Here's the drawing with two shaded views (mm, measured from the low corner). I have some questions. Coordinates: 2 decimals unless noted, no trailing zeros. Order: outer loops, then holes, each group sorted by start corner. A loop starts at its lowest first (then second) coordinate and runs counter-clockwise, first axis right, second up. Notation, with made-up numbers: (89, -8.75) - (102, -8.75) arc R35 ccw to (102, 27.25) - close; hole circle Ø10 at (21, 41). An arc over 180 degrees is marked (long way). Answer as CSV lines item,"result". Start each with the question number.
1. I need wall thicknesses on probe 1 along Y at (x, z) = (6, 100.5); probe 2 along Z at (x, y) = (11.5, 7). Which ranges of each line are inside material? Lowest first, please.
2. I want a section at A-A, the plane x = 6. List the corners of the cut face in (y, z) for me, and give its area (3 significant figures).
3. I want a section at C-C, the plane z = 73. List the corners of the cut face in (x, y) for me, and give its area (3 significant figures).
4. I want a section at B-B, the plane y = 6. List the corners of the cut face in (x, z) for me, and give its area (3 significant figures).
5. I want a section at D-D, the plane y = 10.5. List the corners of the cut face in (x, z) for me, and give its area (3 significant figures).
6. For pin 1 (1.5 mm diameter, centred on x = 5.5, z = 14, fed in from -Y); pin 2 (1.5 mm diameter, centred on x = 10.5, z = 19, fed in from -Y); pin 3 (1.5 mm diameter, centred on y = 7.5, z = 77, fed in from -X); pin 4 (1.5 mm diameter, centred on x = 4, z = 86.5, fed in from -Y), each with a flat end and sliding along its axis, tell me the tip position at first contact or that it passes through.
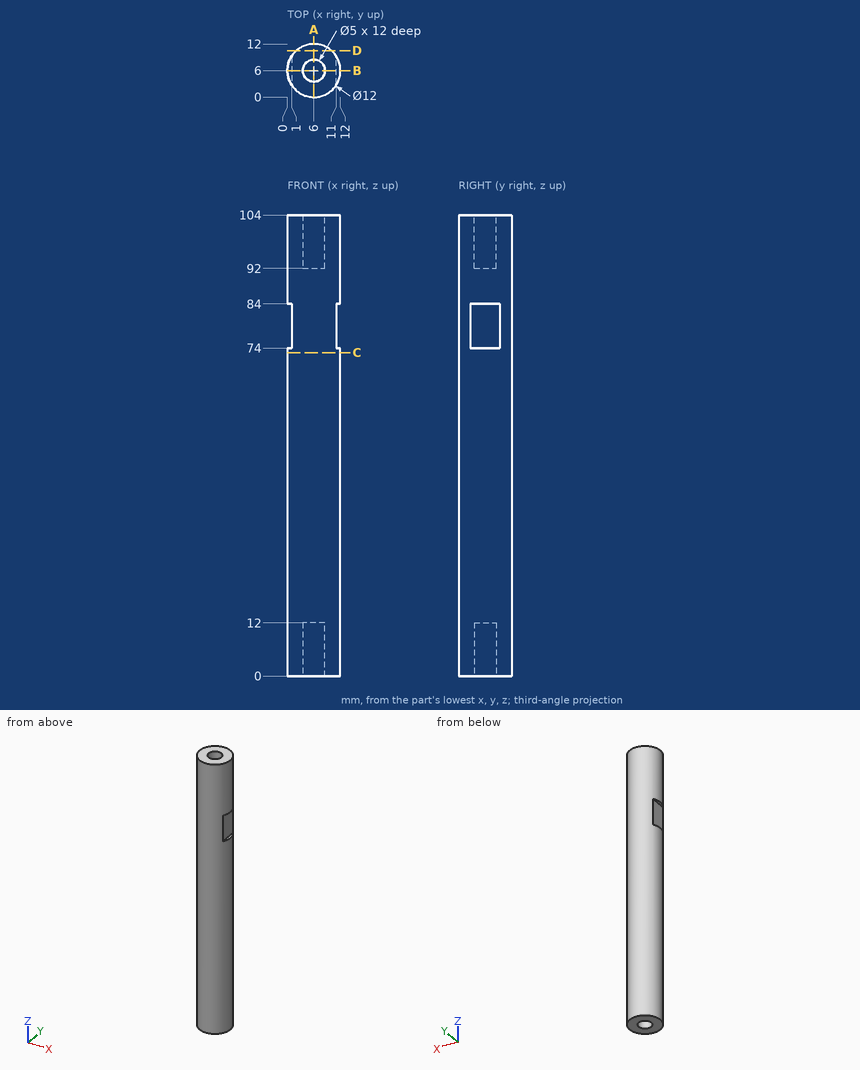
Solved:
1,probe 1,"y = 0 to 3.5, 8.5 to 12"
1,probe 2,"z = 0 to 74, 84 to 104"
2,outline,"(0, 0) - (3.5, 0) - (3.5, 12) - (8.5, 12) - (8.5, 0) - (12, 0) - (12, 104) - (8.5, 104) - (8.5, 92) - (3.5, 92) - (3.5, 104) - (0, 104) - close"
2,area,"1,130 mm2"
3,outline,"circle Ø12 at (6, 6)"
3,area,"113 mm2"
4,outline,"(0, 0) - (3.5, 0) - (3.5, 12) - (8.5, 12) - (8.5, 0) - (12, 0) - (12, 74) - (11, 74) - (11, 84) - (12, 84) - (12, 104) - (8.5, 104) - (8.5, 92) - (3.5, 92) - (3.5, 104) - (0, 104) - (0, 84) - (1, 84) - (1, 74) - (0, 74) - close"
4,area,"1,110 mm2"
5,outline,"(2.03, 0) - (9.97, 0) - (9.97, 104) - (2.03, 104) - close"
5,area,"825 mm2"
6,pin 1,"stops at y = 0"
6,pin 2,"stops at y = 1.32"
6,pin 3,"stops at x = 1"
6,pin 4,"stops at y = 0.13"
